Part model, mm, in its own coordinate system. Give positions to 0.01 mm unless a question says otherwise; leave off trailing zeros. Loops run counter-clockwise (first coordinate to the right, second up) from the corner with the lowest first, then second, coordinate; pieces in that order, holes last. Notation, with made-up numbers: M 73.25,40.5 L 115.25,40.5 A21 cw 115.25,47.5 Z; hole C 7,4.5 d2. An arc over 180 degrees is marked long. Answer in a Markdown table with one row per item.
from build123d import *

# Parameters (mm, degrees)
SKETCH1_R           = 75
BOSS_EXTRUDE1_DEPTH = 50
FILLET1_R           = 8
SKETCH2_R           = 1.5
CUT_EXTRUDE1_DEPTH  = 4


with BuildPart() as part:
    # Sketch1 → Boss-Extrude1 (new body)
    with BuildSketch(Plane(origin=(0, 0, 0), x_dir=(1, 0, 0), z_dir=(0, 1, 0))):
        with Locations(Location((0, 0, 0), (0, 0, 270))):
            Circle(SKETCH1_R)
    extrude(amount=BOSS_EXTRUDE1_DEPTH)

    # Fillet1
    fillet1_edges = [part.edges().sort_by_distance(p)[0] for p in [
        (0, 50, -75),
    ]]
    fillet(fillet1_edges, radius=FILLET1_R)

    # Sketch2 → Cut-Extrude1 (cut)
    with BuildSketch(Plane(origin=(0, 50, 0), x_dir=(1, 0, 0), z_dir=(0, 1, 0))):
        with Locations(Location((0, 13, 0), (0, 0, 270))):
            Circle(SKETCH2_R)
        with Locations(Location((13, 0, 0), (0, 0, 270))):
            Circle(SKETCH2_R)
        with Locations(Location((0, -13, 0), (0, 0, 270))):
            Circle(SKETCH2_R)
        with Locations(Location((-13, 0, 0), (0, 0, 270))):
            Circle(SKETCH2_R)
    extrude(amount=-CUT_EXTRUDE1_DEPTH, mode=Mode.SUBTRACT)


solid = part.part
(1) Drill centre lines: line 1 along X through (y, z) = (49.1, 0); line 2 along Z through (x, y) = (-0.5, 27.5); line 3 along X through (y, z) = (30, -5). Where is each one in solid material? Low to high.
Recorded:
| item | result |
|---|---|
| line 1 | x = -70.69 to -14.5, -11.5 to 11.5, 14.5 to 70.69 |
| line 2 | z = -75 to 75 |
| line 3 | x = -74.83 to 74.83 |
(2) Pin check, flat tips, straight feed: pin 1 Ø0.9 at (x, z) = (0.5, -13) entering from +Y; pin 2 Ø6 at (y, z) = (24.5, 5.5) entering from -X; pin 3 Ø1 at (y, z) = (21.5, 46) entering from -X. Stop position of each tip, or through.
Recorded:
| item | result |
|---|---|
| pin 1 | stops at y = 46 |
| pin 2 | stops at x = -74.96 |
| pin 3 | stops at x = -59.62 |
(3) Saw through at A-A (y = 40). Write the cut outline in (x, z).
Recorded:
| item | result |
|---|---|
| outline | C 0,0 d150 |
